For this review, take the finished solid that the model builds, in its own axes (mm). Face numbers are marked on the shaded views. A direction names the side the tool comes from. Coordinates: 2 decimals unless noted, no trailing zeros. Order: outer loops, then holes, each group sorted by start corner. A loop starts at its lowest first (then second) coordinate and runs counter-clockwise, first axis right, second up. Notation, with made-up numbers: (84.25, -28.5) -> (123.25, -28.5) arc R18 ccw to (123.25, -22.5) -> close; hole circle Ø11 at (14.5, 54.25). An arc over 180 degrees is marked (long way). Answer as a JSON object with one key per item and string values. Group by question number.
1) Machinability: for the marked faces 4 and 5, which of the approach directions +Z, -Z, +X, -X, +Y, -Y give a long, thin tool a straight path to every point of the face, cutting with its end or side? Answer none if there is none.
2) Add section A-A, the plane y = 100.5. Write out the cut boundary in (x, z), then the cut area to 3 significant figures.
3) Wall thickness on L1, parallel to Y at x = 87, z = 12.75; L2, parallel to X at y = 93, z = 15.5: over which ranges is each line inside the solid? List them lowest first.
4) Add section B-B, the plane x = 36. Write out the cut boundary in (y, z).
5) For pin 1 (3 mm diameter, centred on y = 106.5, z = 21, fed in from -X); pin 2 (2 mm diameter, centred on x = 90.93, y = 77.52, fed in from +Z), all flat-tipped, find the tip position at first contact; note any pin that passes through.
6) Draft analysis for pull direction Y (two halves, no side actions). For the marked faces 1, 2 and 3, state which applies: +Y half, -Y half, draft (parallel to the pull), parting line (faces both ways), or undercut.
7) Add section C-C, the plane z = 2.5. Write out the cut boundary in (x, y).
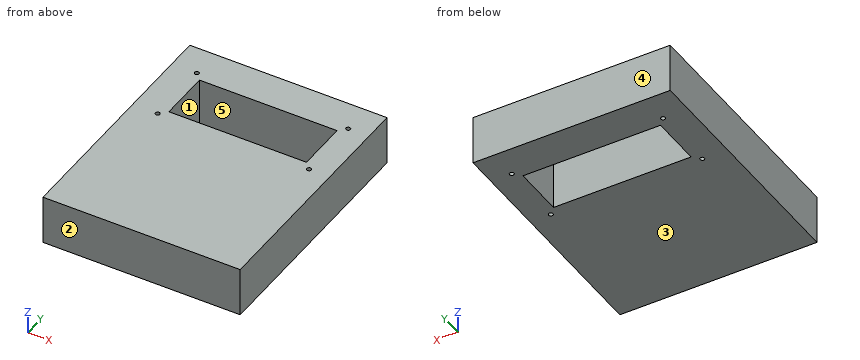
Autodesk Inventor part; units mm, degrees
ref_plane "YZ Plane" through (0, 0, 0) normal (1, 0, 0) x (0, 1, 0)
ref_plane "XZ Plane" through (0, 0, 0) normal (0, 1, 0) x (-1, 0, 0)
ref_plane "XY Plane" through (0, 0, 0) normal (0, 0, 1) x (1, 0, 0)
sketch "Sketch1" plane through (0, 0, 0) normal (0, 0, 1) x (1, 0, 0)
  line L0 (0, 0) -> (101.6, 0)
  line L1 (101.6, 0) -> (101.6, 127)
  line L2 (101.6, 127) -> (0, 127)
  line L3 (0, 127) -> (0, 0)
  line L4 (0, 127) -> (10.668, 127)
  line L5 (101.6, 127) -> (90.932, 127)
  circle A0 centre (90.932, 77.5208) radius 1.1303
  line L6 (87.376, 81.2292) -> (16.4846, 81.2292)
  line L7 (16.4846, 81.2292) -> (16.4846, 107.6706)
  line L8 (16.4846, 107.6706) -> (87.376, 107.6706)
  line L9 (87.376, 107.6706) -> (87.376, 81.2292)
  circle A1 centre (12.9286, 111.379) radius 1.1303
  circle A2 centre (12.9286, 77.5208) radius 1.1303
  circle A3 centre (90.932, 111.379) radius 1.1303
  line L10 (0, 0) -> (12.7, 0)
  line L11 (12.7, 0) -> (12.7, -4.064)
  line L12 (12.7, -4.064) -> (0, -4.064)
  line L13 (0, -4.064) -> (0, 0)
  line L14 (25.4, -4.064) -> (38.1, -4.064)
  line L15 (38.1, -4.064) -> (38.1, 0)
  line L16 (38.1, 0) -> (25.4, 0)
  line L17 (25.4, 0) -> (25.4, -4.064)
  line L18 (50.8, -4.064) -> (63.5, -4.064)
  line L19 (63.5, -4.064) -> (63.5, 0)
  line L20 (63.5, 0) -> (50.8, 0)
  line L21 (50.8, 0) -> (50.8, -4.064)
  line L22 (76.2, -4.064) -> (88.9, -4.064)
  line L23 (88.9, -4.064) -> (88.9, 0)
  line L24 (88.9, 0) -> (76.2, 0)
  line L25 (76.2, 0) -> (76.2, -4.064)
  line L26 (12.7, 127) -> (12.7, 131.064)
  line L27 (12.7, 131.064) -> (0, 131.064)
  line L28 (0, 131.064) -> (0, 127)
  line L29 (25.4, 131.064) -> (38.1, 131.064)
  line L30 (38.1, 131.064) -> (38.1, 127)
  line L31 (25.4, 127) -> (25.4, 131.064)
  line L32 (50.8, 131.064) -> (63.5, 131.064)
  line L33 (63.5, 131.064) -> (63.5, 127)
  line L34 (50.8, 127) -> (50.8, 131.064)
  line L35 (76.2, 131.064) -> (88.9, 131.064)
  line L36 (88.9, 131.064) -> (88.9, 127)
  line L37 (76.2, 127) -> (76.2, 131.064)
  dimension "d0" = 101.6
  dimension "d1" = 127
  dimension "d2" = 10.668
  dimension "d3" = 10.668
  dimension "d7" = 2.2606
  dimension "d23" = 2.2606
  dimension "d24" = 2.2606
  dimension "d25" = 2.2606
  dimension "d28" = 12.7
  dimension "d29" = 4.064
  dimension "d30" = 12.7
  dimension "d31" = 12.7
  dimension "d32" = 12.7
  dimension "d33" = 12.7
  dimension "d34" = 12.7
  dimension "d35" = 12.7
extrude "Extrusion1" add sketch "Sketch1" along normal blind 25.4 contours L3 L2 L1 L0
properties part number "ProtoFront"
Output values:
{
 "1": {"face 4": "+Z, -Z, +X, -X, +Y", "face 5": "+Z, -Z"},
 "2": {"outline": "(0, 0) -> (16.48, 0) -> (16.48, 25.4) -> (0, 25.4) -> close; (87.38, 0) -> (101.6, 0) -> (101.6, 25.4) -> (87.38, 25.4) -> close", "area": "780 mm²"},
 "3": {"L1": "y = 0 to 81.23, 107.67 to 127", "L2": "x = 0 to 16.48, 87.38 to 101.6"},
 "4": {"outline": "(0, 0) -> (81.23, 0) -> (81.23, 25.4) -> (0, 25.4) -> close; (107.67, 0) -> (127, 0) -> (127, 25.4) -> (107.67, 25.4) -> close"},
 "5": {"pin 1": "stops at x = 0", "pin 2": "passes through"},
 "6": {"face 1": "undercut", "face 2": "-Y half", "face 3": "draft"},
 "7": {"outline": "(0, 0) -> (101.6, 0) -> (101.6, 127) -> (0, 127) -> close; hole circle Ø2.26 at (12.93, 77.52); hole circle Ø2.26 at (12.93, 111.38); hole (16.48, 81.23) -> (87.38, 81.23) -> (87.38, 107.67) -> (16.48, 107.67) -> close; hole circle Ø2.26 at (90.93, 77.52); hole circle Ø2.26 at (90.93, 111.38)"}
}
